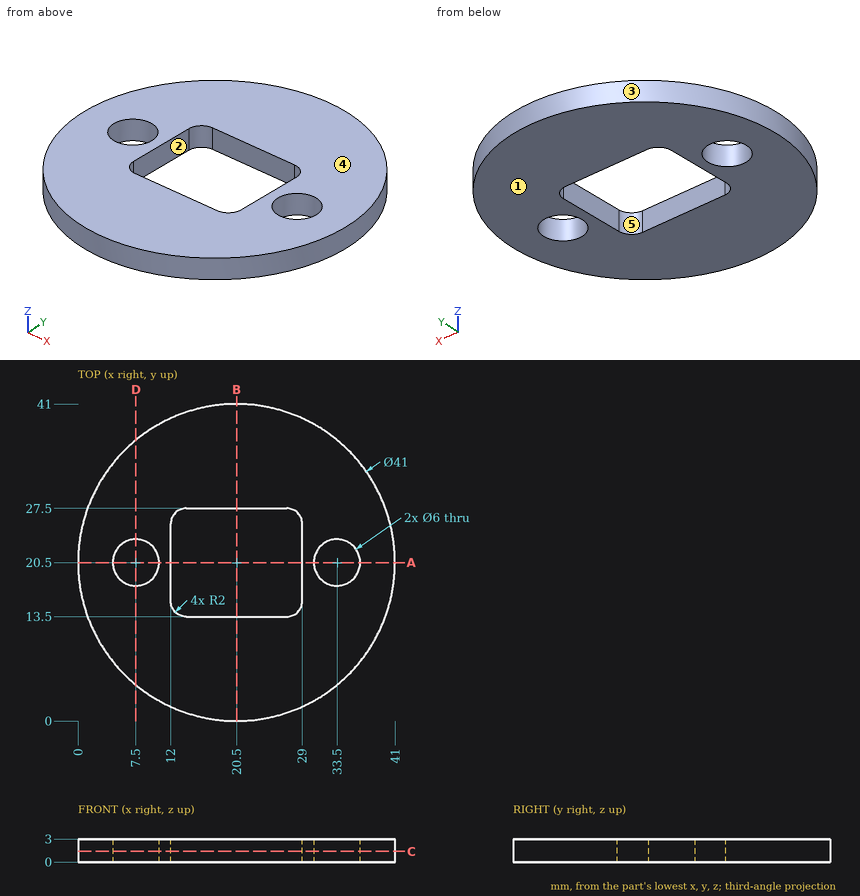
Answer from the drawing. Dimensions are ordinates in mm from the lowest x, y and z of the part. A direction names the side the tool comes from. Coordinates: 2 decimals unless noted, no trailing zeros. Order: outer loops, then holes, each group sorted by start corner. A loop starts at its lowest first (then second) coordinate and runs counter-clockwise, first axis right, second up. Notation, with made-up numbers: (53.5, 5.25) -> (67.5, 5.25) arc R38 ccw to (67.5, 43.25) -> close; hole circle Ø1 at (-37.5, 14.5). An arc over 180 degrees is marked (long way). Answer as a JSON object with one key per item and string values.
1) A cutting plane is placed at D-D, the plane x = 7.5. Determine the outline of the cut face in (y, z).
Model answer:
{"outline": "(4.65, 0) -> (17.5, 0) -> (17.5, 3) -> (4.65, 3) -> close; (23.5, 0) -> (36.35, 0) -> (36.35, 3) -> (23.5, 3) -> close"}
2) A tool of negligible diameter and unlimited length cuts with its end or side. For the marked faces 4 and 5, from which of +Z, -Z, +X, -X, +Y, -Y can it reach the whole face along a straight path? Write none if from no direction.
Model answer:
{"face 4": "+Z, +X, -X, +Y, -Y", "face 5": "+Z, -Z"}
3) A cutting plane is placed at A-A, the plane y = 20.5. Determine the outline of the cut face in (x, z).
Model answer:
{"outline": "(0, 0) -> (4.5, 0) -> (4.5, 3) -> (0, 3) -> close; (10.5, 0) -> (12, 0) -> (12, 3) -> (10.5, 3) -> close; (29, 0) -> (30.5, 0) -> (30.5, 3) -> (29, 3) -> close; (36.5, 0) -> (41, 0) -> (41, 3) -> (36.5, 3) -> close"}
4) A cutting plane is placed at B-B, the plane x = 20.5. Determine the outline of the cut face in (y, z).
Model answer:
{"outline": "(0, 0) -> (13.5, 0) -> (13.5, 3) -> (0, 3) -> close; (27.5, 0) -> (41, 0) -> (41, 3) -> (27.5, 3) -> close"}
5) A cutting plane is placed at C-C, the plane z = 1.4. Determine the outline of the cut face in (x, y).
Model answer:
{"outline": "circle Ø41 at (20.5, 20.5); hole circle Ø6 at (7.5, 20.5); hole (12, 15.5) arc R2 ccw to (14, 13.5) -> (27, 13.5) arc R2 ccw to (29, 15.5) -> (29, 25.5) arc R2 ccw to (27, 27.5) -> (14, 27.5) arc R2 ccw to (12, 25.5) -> close; hole circle Ø6 at (33.5, 20.5)"}
6) Each of these flat-tipped pins is pushed along its axis until it touches: pin 1 (5 mm diameter, centred on x = 33.5, y = 20.5, fed in from +Z); pin 2 (1.5 mm diameter, centred on x = 22.5, z = 2, fed in from +Y); pin 3 (0.9 mm diameter, centred on y = 19.5, z = 1.5, fed in from +X). Where does it stop, or does it pass through?
Model answer:
{"pin 1": "passes through", "pin 2": "stops at y = 40.96", "pin 3": "stops at x = 40.99"}
7) The mould has two halves that part along Y. Classify the marked faces 1, 2 and 3: released by +Y, released by -Y, zero draft, split by the parting line, or undercut.
Model answer:
{"face 1": "zero draft", "face 2": "undercut", "face 3": "split by the parting line"}
8) Consider line 1 along Y through (x, z) = (21, 1.25); line 2 along Y through (x, z) = (14, 0.15); line 3 along X through (y, z) = (25, 1.65). Determine where each line is inside the solid, lowest interval first. Write a range as from..to.
Model answer:
{"line 1": "y = 0.01..13.5, 27.5..40.99", "line 2": "y = 1.06..13.5, 27.5..39.94", "line 3": "x = 0.5..12, 29..40.5"}
